Here's how the part is built. I have some questions about the finished solid (model axes, mm). Give positions to 0.01 mm unless a question says otherwise; leave off trailing zeros. Write each loop counter-clockwise with the first axis right and the second up, starting at its lowest first coordinate (ties: lowest second). Pieces come first, ordered by that corner, then holes. Notation, with made-up numbers: (72, 73) -> (86, 73) arc R30 ccw to (86, 112) -> close; hole circle Ø2 at (48, 54). An arc over 180 degrees is marked (long way). Return JSON: item names as keys, results as strings.
from build123d import *

# Parameters (mm, degrees)
F0_R     = 51.217295
F0_R_2   = 40.297185
F1_DEPTH = 25.4
F2_R     = 5.08
F3_R     = 5.08
F4_R     = 5.08


with BuildPart() as f1:
    # F0 (on Front) → F1 (new body)
    with BuildSketch(Plane.XZ):
        with Locations((-93.010761, 45.482028)):
            Circle(F0_R)
        with Locations((-93.010761, 45.482028)):
            Circle(F0_R_2, mode=Mode.SUBTRACT)
    extrude(amount=F1_DEPTH)

    # F2
    f2_edges = [f1.edges().sort_by_distance(p)[0] for p in [
        (-144.228056, -25.4, 45.482028),
        (-144.228056, 0, 45.482028),
    ]]
    fillet(f2_edges, radius=F2_R)

    # F3
    f3_edges = [f1.edges().sort_by_distance(p)[0] for p in [
        (-133.307946, -25.4, 45.482028),
    ]]
    fillet(f3_edges, radius=F3_R)

    # F4
    f4_edges = [f1.edges().sort_by_distance(p)[0] for p in [
        (-133.307946, 0, 45.482028),
    ]]
    fillet(f4_edges, radius=F4_R)


solid = f1.part
1. Suppose I cut it at A-A, the plane y = -2.75. List the corners of the cut face in (x, z) for me.
Taken from the geometry:
{"outline": "circle Ø101.3 at (-93.01, 45.48); hole circle Ø81.73 at (-93.01, 45.48)"}
2. For pin 1 Ø12 at (y, z) = (-18.5, 84.5) entering from +X; pin 2 Ø8 at (x, y) = (-59.5, -10.5) entering from -Z; pin 3 Ø4 at (y, z) = (-8, 10) entering from -X, each with a flat end and sliding along its axis, tell me the tip position at first contact or that it passes through.
Taken from the geometry:
{"pin 1": "stops at x = -53.86", "pin 2": "stops at z = 3.62", "pin 3": "stops at x = -131.77"}
3. If I drill on line 1 (X direction, y = -12.5, z = 43); line 2 (X direction, y = -8.25, z = 64.5); line 3 (Z direction, x = -69.5, y = -15.5), over which ranges is the centre line in solid material (lowest first)? Write a range as [from, to].
Taken from the geometry:
{"line 1": "x = [-144.17, -133.23], [-52.79, -41.85]", "line 2": "x = [-140.57, -128.54], [-57.48, -45.46]", "line 3": "z = [-0.02, 12.75], [78.21, 90.98]"}
4. If we mould it in two halves opening along X, with no side actions, what happens to faces 1 (the face through (-99.678, -12.593, 96.263)), 2 (the face through (-59, 0, 15)), 3 (the face through (-101.746, -12.593, 6.143))? For each: released by +X, released by -X, zero draft, split by the parting line, or undercut.
Taken from the geometry:
{"face 1": "split by the parting line", "face 2": "zero draft", "face 3": "undercut"}
